```python
from build123d import *

# Parameters (mm, degrees)
FILLET2_R     = 1
FILLET3_R     = 0.4
CHAMFER1_SIZE = 0.3


with BuildPart() as part:
    # Sketch1 → Revolve1 (revolve)
    with BuildSketch(Plane.XY, mode=Mode.PRIVATE) as revolve1_sk:
        Polygon((2.75, 0), (2.75, 1.4), (5, 1.4), (5, 3), (6, 3), (10, 1.544119063), (10, 0), align=None)
    revolve(revolve1_sk.sketch.rotate(Axis((0, 0, 0), (0, 1, 0)), 90), axis=Axis((0, 0, 0), (0, 1, 0)))

    # Fillet2
    fillet2_edges = [part.edges().sort_by_distance(p)[0] for p in [
        (0, 1.544119063, 10),
    ]]
    fillet(fillet2_edges, radius=FILLET2_R)

    # Fillet3
    fillet3_edges = [part.edges().sort_by_distance(p)[0] for p in [
        (0, 1.4, 5),
    ]]
    fillet(fillet3_edges, radius=FILLET3_R)

    # Chamfer1
    chamfer1_edges = [part.edges().sort_by_distance(p)[0] for p in [
        (0, 0, 10),
        (0, 1.4, 2.75),
        (0, 0, 2.75),
    ]]
    chamfer(chamfer1_edges, length=CHAMFER1_SIZE)


solid = part.part
```
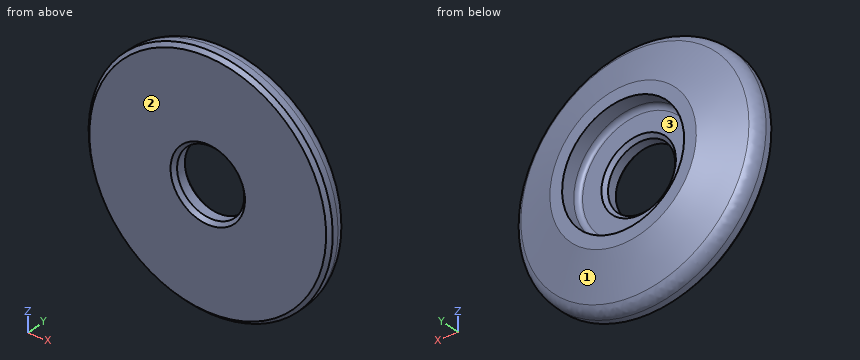
The model under review builds one solid part; all positions refer to its coordinate system, in mm. Face numbers are marked on the shaded views. Round coordinates to 2 decimals unless told otherwise and drop trailing zeros. Loops run counter-clockwise (first coordinate to the right, second up) from the corner with the lowest first, then second, coordinate; pieces in that order, holes last. Notation, with made-up numbers: (-20.5, -9) - (38.5, -9) arc R35 ccw to (38.5, 23) - close; hole circle Ø6 at (55.5, 89). An arc over 180 degrees is marked (long way). Use a Markdown table: item, result. Add a question column.
Q1. Add section A-A (y = 0.6). State the section outline as (x, z) points, plus the area to 3 significant figures.
Q2. For probe 1 along X at (y, z) = (0.85, 0); probe 2 along X at (y, z) = (1.6, 1.25); probe 3 along Z at (x, y) = (1, 1.75), list the stretches that pass through material, from the lowest coordinate up.
Q3. Insertion check: pin 1 Ø1 at (x, y) = (4, 0.5) entering from +Z; pin 2 Ø6.5 at (x, z) = (0, 0) entering from +Y; pin 3 Ø1 at (y, z) = (1.5, -3.5) entering from +X. Each pin has a flat end and moves straight along its axis. Give the tip position at first contact, or say it passes through.
Q4. The part is to be moulded in two halves that separate along X. For the marked faces 1, 2 and 3, say which applies: pulls with the +X half, pulls with the -X half, needs draft (parallel to the pull), parting line crosses it, or undercut.
Q5. Add section B-B (y = 2.55). State the section outline as (x, z) points.
Worked answers:
| question | item | result |
|---|---|---|
| 1 | outline | circle Ø20 at (0, 0); hole circle Ø5.5 at (0, 0) |
| 1 | area | 290 mm² |
| 2 | probe 1 | -10 to -2.75, 2.75 to 10 |
| 2 | probe 2 | -9.57 to -4.79, 4.79 to 9.57 |
| 2 | probe 3 | -9.37 to -4.9, 4.9 to 9.37 |
| 3 | pin 1 | z = 9.37 |
| 3 | pin 2 | y = 1.4 |
| 3 | pin 3 | x = 9.44 |
| 4 | face 1 | parting line crosses it |
| 4 | face 2 | needs draft |
| 4 | face 3 | undercut |
| 5 | outline | circle Ø14.47 at (0, 0); hole circle Ø10 at (0, 0) |
